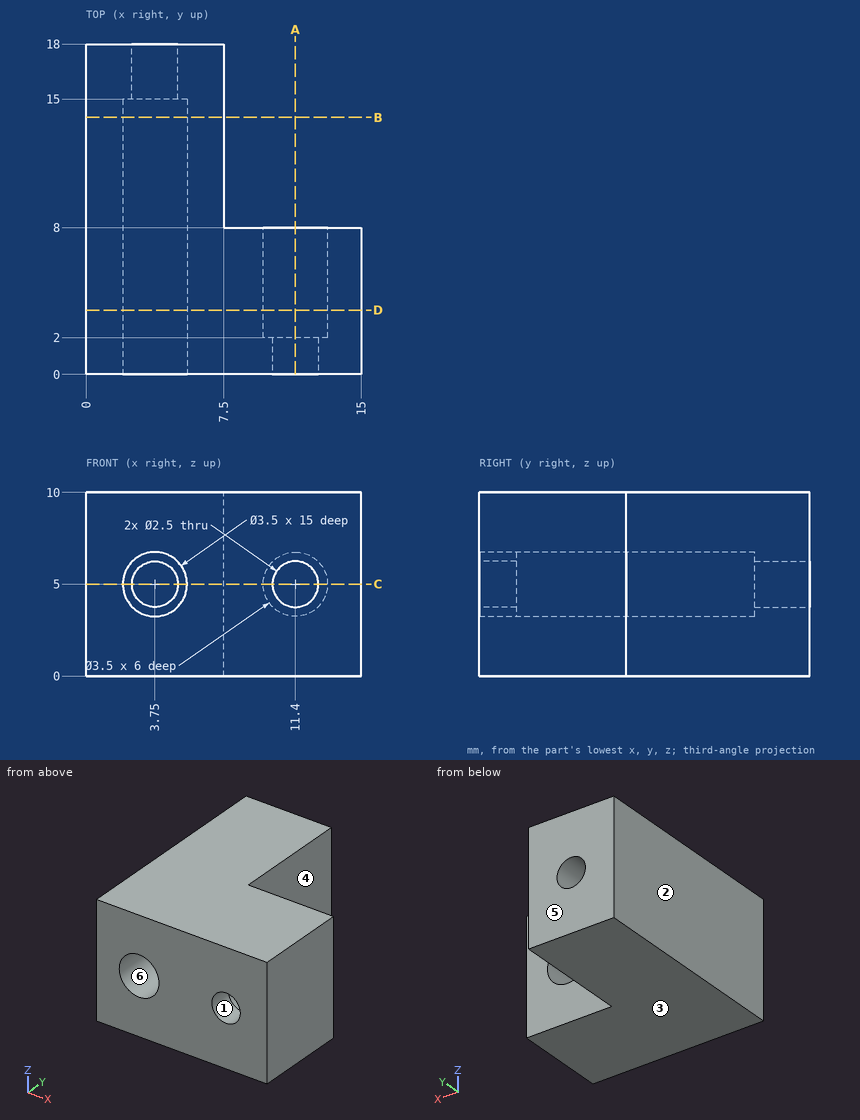
For this review, use the dimensioned drawing (mm, ordinates from the lowest corner) and the shaded views. A direction names the side the tool comes from. Coordinates: 2 decimals unless noted, no trailing zeros. Write each loop counter-clockwise with the first axis right and the second up, starting at its lowest first coordinate (ties: lowest second). Pieces come first, ordered by that corner, then holes. Notation, with made-up numbers: (81.5, -8) - (119.5, -8) arc R25 cw to (119.5, 22) - close; hole circle Ø1 at (21, -1.5). An arc over 180 degrees is marked (long way). Answer as a JSON object with one key per item and string values. Group by question number.
1. Mouldability with a two-part tool opening along Z and no side actions: class the marked faces 1, 2 and 3 as pulls with the +Z half, pulls with the -Z half, needs draft (parallel to the pull), parting line crosses it, or undercut.
2. To check wall thickness, follow probe 1 along X at (y, z) = (3.2, 5); probe 2 along Y at (x, z) = (10.5, 0.5); probe 3 along Z at (x, y) = (11.4, 0.85). State the ranges of each line that lie inside material, in increasing order.
3. Add section A-A (x = 11.4). Give the boundary of the cut face in (y, z), plus the area to 3 significant figures.
4. Machinability: for the marked faces 4, 5 and 6, which of the approach directions +Z, -Z, +X, -X, +Y, -Y give a long, thin tool a straight path to every point of the face, cutting with its end or side? Answer none if there is none.
5. Add section C-C (z = 5). Give the boundary of the cut face in (x, y), plus the area to 3 significant figures.
6. Add section B-B (y = 14). Give the boundary of the cut face in (x, z).
7. Clearance check with flat-ended pins moving along their axes: pin 1 Ø1.8 at (x, z) = (11.5, 6) entering from +Y; pin 2 Ø2 at (x, z) = (11.4, 5) entering from +Y. State where each tip first meets the part, or that it passes through.
8. Add section D-D (y = 3.5). Give the boundary of the cut face in (x, z), plus the area to 3 significant figures.
Findings:
{
 "1": {"face 1": "undercut", "face 2": "needs draft", "face 3": "pulls with the -Z half"},
 "2": {"probe 1": "0 to 2, 5.5 to 9.65, 13.15 to 15", "probe 2": "0 to 8", "probe 3": "0 to 3.75, 6.25 to 10"},
 "3": {"outline": "(0, 0) - (8, 0) - (8, 3.25) - (2, 3.25) - (2, 3.75) - (0, 3.75) - close; (0, 6.25) - (2, 6.25) - (2, 6.75) - (8, 6.75) - (8, 10) - (0, 10) - close", "area": "54.0 mm²"},
 "4": {"face 4": "+Z, -Z, +X, +Y", "face 5": "+Z, -Z, +X, -X, +Y", "face 6": "-Y"},
 "5": {"outline": "(0, 0) - (2, 0) - (2, 15) - (2.5, 15) - (2.5, 18) - (0, 18) - close; (5, 15) - (5.5, 15) - (5.5, 0) - (10.15, 0) - (10.15, 2) - (9.65, 2) - (9.65, 8) - (7.5, 8) - (7.5, 18) - (5, 18) - close; (12.65, 0) - (15, 0) - (15, 8) - (13.15, 8) - (13.15, 2) - (12.65, 2) - close", "area": "109 mm²"},
 "6": {"outline": "(0, 0) - (7.5, 0) - (7.5, 10) - (0, 10) - close; hole circle Ø3.5 at (3.75, 5)"},
 "7": {"pin 1": "y = 8", "pin 2": "through"},
 "8": {"outline": "(0, 0) - (15, 0) - (15, 10) - (0, 10) - close; hole circle Ø3.5 at (3.75, 5); hole circle Ø3.5 at (11.4, 5)", "area": "131 mm²"}
}
